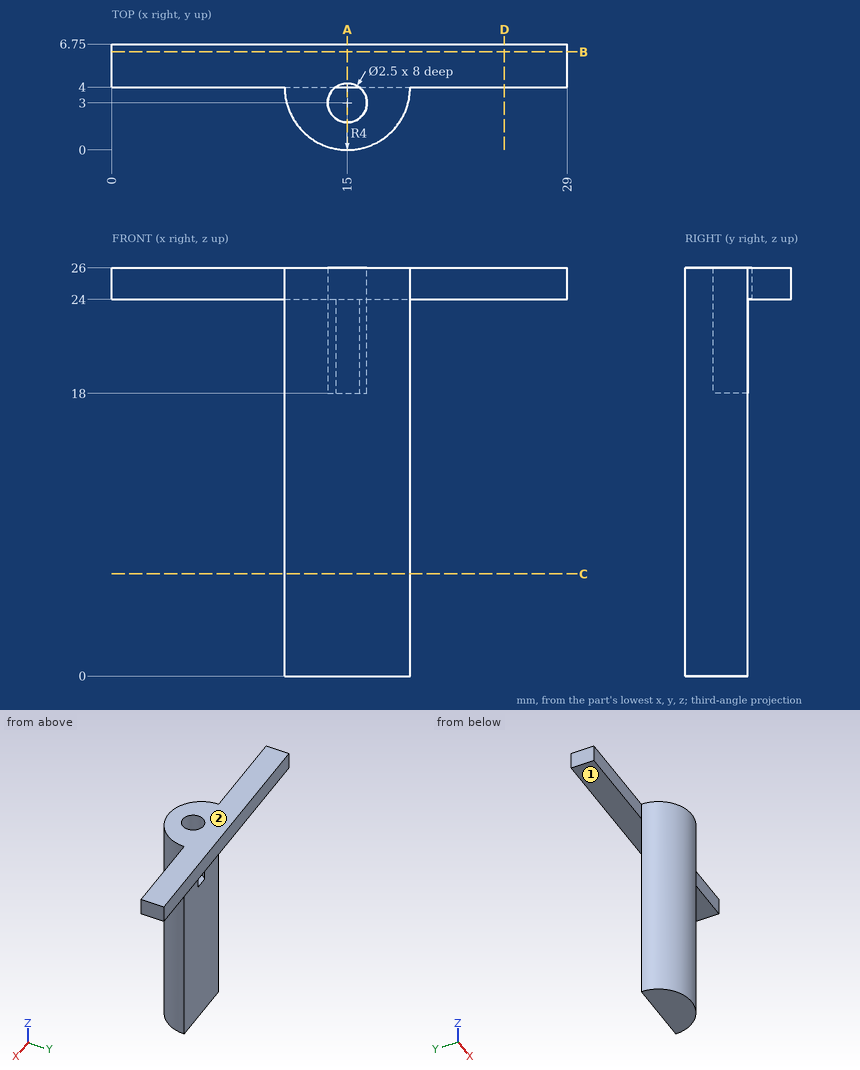
For this review, use the dimensioned drawing (mm, ordinates from the lowest corner) and the shaded views. A direction names the side the tool comes from. Round coordinates to 2 decimals unless told otherwise and drop trailing zeros. Write each loop counter-clockwise with the first axis right and the second up, starting at its lowest first coordinate (ties: lowest second). Pieces come first, ordered by that corner, then holes. Notation, with made-up numbers: (51.25, -9) - (62.25, -9) arc R25 cw to (62.25, 18) - close; hole circle Ø7 at (64, -29). An arc over 180 degrees is marked (long way). Answer as a JSON object with one key per item and string values.
1. We need section C-C on z = 6.5. Give the boundary of the cut face in (x, y).
Response values:
{"outline": "(11, 4) arc R4 ccw to (19, 4) - close"}
2. Tool access review of the marked faces 1 and 2: name each direction out of +Z, -Z, +X, -X, +Y, -Y from which nothing blocks a thin tool from reaching the whole face with its end or side.
Response values:
{"face 1": "-Z, +X, -X, +Y", "face 2": "+Z, +X, -X, +Y, -Y"}
3. We need section A-A on x = 15. Give the boundary of the cut face in (y, z).
Response values:
{"outline": "(0, 0) - (4, 0) - (4, 18) - (1.75, 18) - (1.75, 26) - (0, 26) - close; (4.25, 24) - (6.75, 24) - (6.75, 26) - (4.25, 26) - close"}
4. We need section B-B on y = 6.25. Give the boundary of the cut face in (x, z).
Response values:
{"outline": "(0, 24) - (29, 24) - (29, 26) - (0, 26) - close"}
5. For pin 1 Ø4 at (x, z) = (15, 14) entering from +Y; pin 2 Ø2 at (x, y) = (9.5, 6) entering from -Z; pin 3 Ø0.6 at (x, z) = (5.5, 25) entering from -Y, all flat-tipped, find the tip position at first contact; note any pin that passes through.
Response values:
{"pin 1": "stops at y = 4", "pin 2": "stops at z = 24", "pin 3": "stops at y = 4"}
6. To check wall thickness, follow line 1 along Y through (x, z) = (15, 24.25); line 2 along Z through (x, y) = (20, 5.75); line 3 along Y through (x, z) = (7, 24.5). State the ranges of each line that lie inside material, in increasing order.
Response values:
{"line 1": "y = 0 to 1.75, 4.25 to 6.75", "line 2": "z = 24 to 26", "line 3": "y = 4 to 6.75"}
7. We need section D-D on x = 25. Give the boundary of the cut face in (y, z), then the cut area to 3 significant figures.
Response values:
{"outline": "(4, 24) - (6.75, 24) - (6.75, 26) - (4, 26) - close", "area": "5.50 mm2"}
